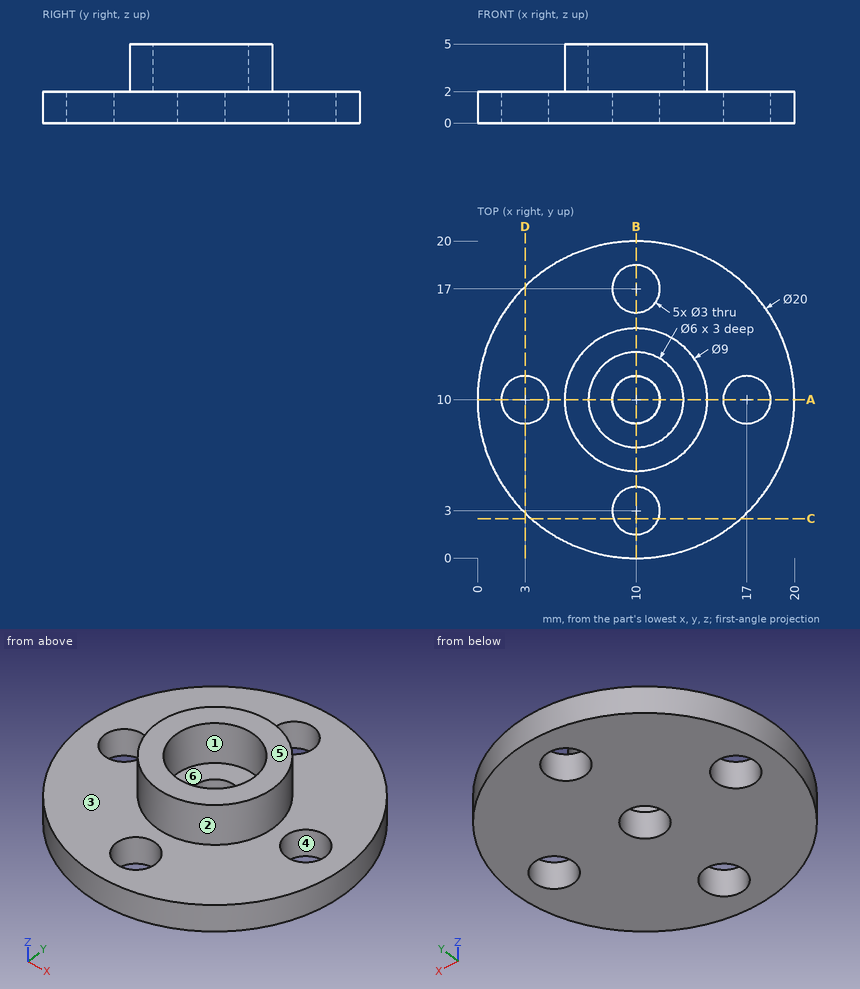
For this review, use the dimensioned drawing (mm, ordinates from the lowest corner) and the shaded views. A direction names the side the tool comes from. Round coordinates to 2 decimals unless told otherwise and drop trailing zeros. Order: outer loops, then holes, each group sorted by start corner. A loop starts at its lowest first (then second) coordinate and runs counter-clockwise, first axis right, second up. Notation, with made-up numbers: M 38.25,28 L 85.25,28 A37 cw 85.25,67 Z; hole C -3.75,69.5 d7. An arc over 180 degrees is marked long. Use a Markdown table: item, result.
1) Draft analysis for pull direction Y (two halves, no side actions). For the marked faces 1, 2, 3 and 4, state which applies: released by +Y, released by -Y, zero draft, split by the parting line, or undercut.
Report:
| item | result |
|---|---|
| face 1 | undercut |
| face 2 | split by the parting line |
| face 3 | zero draft |
| face 4 | undercut |
2) Consider section A-A (y = 10). Write out the cut boundary in (x, z), then the cut area to 3 significant figures.
Report:
| item | result |
|---|---|
| outline | M 0,0 L 1.5,0 L 1.5,2 L 0,2 Z; M 4.5,0 L 8.5,0 L 8.5,2 L 7,2 L 7,5 L 5.5,5 L 5.5,2 L 4.5,2 Z; M 11.5,0 L 15.5,0 L 15.5,2 L 14.5,2 L 14.5,5 L 13,5 L 13,2 L 11.5,2 Z; M 18.5,0 L 20,0 L 20,2 L 18.5,2 Z |
| area | 31.0 mm^2 |
3) Wall thickness on line 1 along Y through (x, z) = (10, 1.6); line 2 along Z through (x, y) = (7.75, 1.5); line 3 along Y through (x, z) = (12.5, 4.55): over which ranges is each line inside the solid? List them lowest first. Write a range as [from, to].
Report:
| item | result |
|---|---|
| line 1 | [0, 1.5], [4.5, 8.5], [11.5, 15.5], [18.5, 20] |
| line 2 | [0, 2] |
| line 3 | [6.26, 8.34], [11.66, 13.74] |
4) Consider section C-C (y = 2.5). Write out the cut boundary in (x, z), then the cut area to 3 significant figures.
Report:
| item | result |
|---|---|
| outline | M 3.39,0 L 8.59,0 L 8.59,2 L 3.39,2 Z; M 11.41,0 L 16.61,0 L 16.61,2 L 11.41,2 Z |
| area | 20.8 mm^2 |
5) Tool access review of the marked faces 5 and 6: name each direction out of +Z, -Z, +X, -X, +Y, -Y from which nothing blocks a thin tool from reaching the whole face with its end or side.
Report:
| item | result |
|---|---|
| face 5 | +Z, +X, -X, +Y, -Y |
| face 6 | +Z |
6) Consider section D-D (x = 3). Write out the cut boundary in (y, z).
Report:
| item | result |
|---|---|
| outline | M 2.86,0 L 8.5,0 L 8.5,2 L 2.86,2 Z; M 11.5,0 L 17.14,0 L 17.14,2 L 11.5,2 Z |
7) Insertion check: pin 1 (3.5 mm diameter, centred on x = 10, y = 3, fed in from +Z); pin 2 (2 mm diameter, centred on y = 8, z = 2, fed in from +X). Each pin has a flat end and moves straight along its axis. Give the tip position at first contact, or say it passes through.
Report:
| item | result |
|---|---|
| pin 1 | z = 2 |
| pin 2 | x = 19.95 |
